Could you check a few things on this model? Use its own coordinates, in mm. A direction names the side the tool comes from. Round coordinates to 2 decimals unless told otherwise and drop trailing zeros. Loops run counter-clockwise (first coordinate to the right, second up) from the corner with the lowest first, then second, coordinate; pieces in that order, holes last. Notation, with made-up numbers: (70, 73.5) -> (78, 73.5) arc R19 cw to (78, 91.5) -> close; hole circle Ø2 at (-1.5, -37.75). An arc over 180 degrees is marked (long way). Put each result on its own line as item: value. Start each with the question number.
1. Imagine slicing it at B-B, the plane x = 11.5. Please give me the cut outline in (y, z).
2. If we mould it in two halves opening along X, with no side actions, what happens to faces 4 (the flat face through (-21, 0, -54)), 5 (the flat face through (-12, 0, 7)), 6 (the flat face through (-28, 0, 9))? For each: pulls with the +X half, pulls with the -X half, needs draft (parallel to the pull), parting line crosses it, or undercut.
3. I'm going to push flat-ended pins straight in: P1, Ø5, axis at x = -24, y = -7, coming from the -Z side; P2, Ø3.5, axis at x = 24, y = 7, coming from the +Z side; P3, Ø1.8, axis at x = -11.5, y = 0, coming from the +Z side; P4, Ø4.5, axis at x = 0, y = 1.5, coming from the -Z side. Where does each tip first touch, or does it pass through?
4. Imagine slicing it at D-D, the plane z = -50. Please give me the cut outline in (x, y).
5. Imagine slicing it at C-C, the plane z = -4. Please give me the cut outline in (x, y), and give its area (3 significant figures).
6. Imagine slicing it at A-A, the plane y = -7. Please give me the cut outline in (x, z), and give its area (3 significant figures).
7. I need wall thicknesses on line 1 (Y direction, x = -24, z = 9.5); line 2 (X direction, y = -1.75, z = 3.5); line 3 (Z direction, x = 16, y = 6). Which ranges of each line are inside material? Lowest first, please. Write a range as [from, to].
8. Which directions (+Z, -Z, +X, -X, +Y, -Y) give clear straight access to the entire face, cutting with the end or side of a thin tool? Please do faces 1 (the flat face through (0, 0, 13)), 2 (the cylindrical face through (-13, 0, 8)), 3 (the cylindrical face through (-0.943, -4.247, -20.39)).
```python
from build123d import *

# Parameters (mm, degrees)
SKETCH_4_R               = 3
EXTRUDE_1_DEPTH          = 54
CUT_EXTRUDE_1_DEPTH      = 63.657800791
SKETCH_6_R               = 4
CUT_EXTRUDE_2_DEPTH      = 4.5
SKETCH_7_R               = 2.25
CUT_EXTRUDE_3_DEPTH      = 21.5
EXTRUDE_2_DEPTH          = 54
SKETCH_9_R               = 2.5
CUT_EXTRUDE_4_DEPTH      = 5
SKETCH_10_R              = 2.5
CUT_EXTRUDE_5_DEPTH      = 5
SKETCH_11_R              = 4.35
CUT_EXTRUDE_6_DEPTH      = 46.5
SKETCH_12_R              = 1.5
CUT_EXTRUDE_7_DEPTH      = 3
SKETCH_13_R              = 1.5
EXTRUDE_4_DEPTH          = 3
SKETCH_14_R              = 1.5
CUT_EXTRUDE_8_DEPTH      = 6
CUT_EXTRUDE_9_DEPTH      = 3
EXTRUDE_START            = 5
SKETCH_16_W              = 56
SKETCH_16_H              = 22
EXTRUDE_5_DEPTH          = 8
SKETCH_18_R              = 3
EXTRUDE_6_DEPTH          = 67
SKETCH_19_R              = 4.35
EXTRUDE_7_DEPTH          = 59.5
SKETCH_20_R              = 2
CUT_EXTRUDE_10_DEPTH     = 8
MIRROR_4_COPY_1_SKETCH_R = 2
MIRROR_4_COPY_1_DEPTH    = 8
CUT_EXTRUDE_START        = -3
SKETCH_21_R              = 1.5
CUT_EXTRUDE_11_DEPTH     = 3
SKETCH_22_R              = 1.5
CUT_EXTRUDE_12_DEPTH     = 3


with BuildPart() as part:
    # 草图4 → 凸台-拉伸1 (new body)
    with BuildSketch(Plane.XY):
        Polygon((-14.75, -7), (-16.25, -7), (-16.25, -6.5), (-20.75, -6.5), (-20.75, -7), (-22.25, -7), (-22.25, -11), (-20.75, -11), (-20.75, -13), (-29, -13), (-29, 13), (-23, 13), (-20.6, 10.6), (-19.1, 10.6), (-16.7, 13), (0, 13), (0, -13), (-16.25, -13), (-16.25, -11), (-14.75, -11), align=None)
        with Locations((-20.5, 0)):
            Circle(SKETCH_4_R, mode=Mode.SUBTRACT)
    extrude(amount=-EXTRUDE_1_DEPTH)

    # 草图5 → 切除-拉伸1 (cut, through all)
    with BuildSketch(Plane.XY):
        Polygon((-5.5, -12), (-4.5, -12), (-4.5, -13), (-2.25, -13), (-2.25, -12), (-1.25, -12), (-1.25, -10), (-5.5, -10), align=None)
    cut_extrude_1 = extrude(amount=-CUT_EXTRUDE_1_DEPTH, mode=Mode.SUBTRACT)

    # 镜向1: 切除-拉伸1 across plane
    add(cut_extrude_1.mirror(Plane.ZX), mode=Mode.SUBTRACT)

    # 草图6 → 切除-拉伸2 (cut)
    with BuildSketch(Plane(origin=(0, 13, 0), x_dir=(-1, 0, 0), z_dir=(0, 1, 0))):
        with Locations(Location((11.5, -25, 0), (0, 0, 90))):
            Circle(SKETCH_6_R)
        with Locations(Location((11.5, -5, 0), (0, 0, 90))):
            Circle(SKETCH_6_R)
    extrude(amount=-CUT_EXTRUDE_2_DEPTH, mode=Mode.SUBTRACT)

    # 草图7 → 切除-拉伸3 (cut)
    with BuildSketch(Plane(origin=(0, 8.5, 0), x_dir=(1, 0, 0), z_dir=(0, 1, 0))):
        with Locations(Location((-11.5, 25, 0), (0, 0, 270))):
            Circle(SKETCH_7_R)
        with Locations(Location((-11.5, 5, 0), (0, 0, 270))):
            Circle(SKETCH_7_R)
    extrude(amount=-CUT_EXTRUDE_3_DEPTH, mode=Mode.SUBTRACT)

    # 镜向2: part across plane


with BuildPart() as part_1:
    add(part.part)
    add(part.part.mirror(Plane(origin=(0, 0, 0), x_dir=(0, 0, 1), z_dir=(1, 0, 0))))

    # 草图8 → 凸台-拉伸2 (add)
    with BuildSketch(Plane.XY):
        Polygon((16.7, 13), (23, 13), (20.6, 10.6), (19.1, 10.6), align=None)
    extrude(amount=-EXTRUDE_2_DEPTH)

    # 草图9 → 切除-拉伸4 (cut)
    with BuildSketch(Plane(origin=(0, 13, 0), x_dir=(1, 0, 0), z_dir=(0, 1, 0))):
        with Locations(Location((18, 46.5, 0), (0, 0, 270))):
            Circle(SKETCH_9_R)
        with Locations(Location((18, 11, 0), (0, 0, 270))):
            Circle(SKETCH_9_R)
    extrude(amount=-CUT_EXTRUDE_4_DEPTH, mode=Mode.SUBTRACT)

    # 草图10 → 切除-拉伸5 (cut)
    with BuildSketch(Plane(origin=(29, 0, 0), x_dir=(0, 0, -1), z_dir=(1, 0, 0))):
        with Locations((11, 8)):
            Circle(SKETCH_10_R)
        with Locations((38.5, 8)):
            Circle(SKETCH_10_R)
    extrude(amount=-CUT_EXTRUDE_5_DEPTH, mode=Mode.SUBTRACT)

    # 草图11 → 切除-拉伸6 (cut)
    with BuildSketch(Plane.XY):
        Circle(SKETCH_11_R)
    extrude(amount=-CUT_EXTRUDE_6_DEPTH, mode=Mode.SUBTRACT)

    # 草图12 → 切除-拉伸7 (cut)
    with BuildSketch(Plane(origin=(0, 0, -54), x_dir=(-1, 0, 0), z_dir=(0, 0, -1))):
        with Locations((-11.5, 0)):
            Circle(SKETCH_12_R)
        with BuildLine():
            Line((11.75, 1.5), (11.25, 1.5))
            ThreePointArc((11.25, 1.5), (9.75, 0), (11.25, -1.5))
            Line((11.25, -1.5), (11.75, -1.5))
            ThreePointArc((11.75, -1.5), (13.25, 0), (11.75, 1.5))
        make_face()
    extrude(amount=-CUT_EXTRUDE_7_DEPTH, mode=Mode.SUBTRACT)

    # 草图13 → 凸台-拉伸4 (add)
    with BuildSketch(Plane(origin=(0, 0, -51), x_dir=(-1, 0, 0), z_dir=(0, 0, -1))):
        with Locations((11.5, 0)):
            Circle(SKETCH_13_R)
        with Locations((-11.5, 0)):
            Circle(SKETCH_13_R)
    extrude(amount=-EXTRUDE_4_DEPTH)

    # 草图14 → 切除-拉伸8 (cut)
    with BuildSketch(Plane.XZ.offset(13)):
        with Locations(Location((-11.5, -15, 0), (0, 0, 270))):
            Circle(SKETCH_14_R)
        with Locations(Location((11.5, -15, 0), (0, 0, 270))):
            Circle(SKETCH_14_R)
    extrude(amount=-CUT_EXTRUDE_8_DEPTH, mode=Mode.SUBTRACT)

    # 草图15 → 切除-拉伸9 (cut)
    with BuildSketch(Plane.XZ.offset(13)):
        with BuildLine():
            Line((-11.75, -13.5), (-11.25, -13.5))
            ThreePointArc((-11.25, -13.5), (-9.75, -15), (-11.25, -16.5))
            Line((-11.25, -16.5), (-11.75, -16.5))
            ThreePointArc((-11.75, -16.5), (-13.25, -15), (-11.75, -13.5))
        make_face()
    extrude(amount=-CUT_EXTRUDE_9_DEPTH, mode=Mode.SUBTRACT)


with BuildPart() as body_2:
    # 草图16 → 凸台-拉伸5 (new body)
    with BuildSketch(Plane.XY.offset(EXTRUDE_START)):
        Rectangle(SKETCH_16_W, SKETCH_16_H)
    extrude(amount=EXTRUDE_5_DEPTH)

    # 草图18 → 凸台-拉伸6 (add)
    with BuildSketch(Plane.XY.offset(13)):
        with Locations((20.5, 0)):
            Circle(SKETCH_18_R)
        with Locations((-20.5, 0)):
            Circle(SKETCH_18_R)
    extrude(amount=-EXTRUDE_6_DEPTH)

    # 草图19 → 凸台-拉伸7 (add)
    with BuildSketch(Plane.XY.offset(13)):
        Circle(SKETCH_19_R)
    extrude(amount=-EXTRUDE_7_DEPTH)

    # 草图20 → 切除-拉伸10 (cut)
    with BuildSketch(Plane.XY.offset(13)):
        with Locations((-24, 7)):
            Circle(SKETCH_20_R)
    cut_extrude_10 = extrude(amount=-CUT_EXTRUDE_10_DEPTH, mode=Mode.SUBTRACT)

    # 镜向3: 切除-拉伸10 across plane
    add(cut_extrude_10.mirror(Plane.ZX), mode=Mode.SUBTRACT)

    # 镜向4: 切除-拉伸10 across plane
    add(cut_extrude_10.mirror(Plane(origin=(0, 0, 0), x_dir=(0, 0, 1), z_dir=(1, 0, 0))), mode=Mode.SUBTRACT)

    # 镜向4 copy 1 sketch → 镜向4 copy 1 (cut)
    with BuildSketch(Plane(origin=(0, 0, 13), x_dir=(-1, 0, 0), z_dir=(0, 0, 1))):
        with Locations((-24, 7)):
            Circle(MIRROR_4_COPY_1_SKETCH_R)
    extrude(amount=-MIRROR_4_COPY_1_DEPTH, mode=Mode.SUBTRACT)

    # 草图21 → 切除-拉伸11 (cut)
    with BuildSketch(Plane.XY.offset(13).offset(CUT_EXTRUDE_START)):
        with Locations((11.5, 0)):
            Circle(SKETCH_21_R)
        with BuildLine():
            Line((-11.75, 1.5), (-11.25, 1.5))
            ThreePointArc((-11.25, 1.5), (-9.75, 0), (-11.25, -1.5))
            Line((-11.25, -1.5), (-11.75, -1.5))
            ThreePointArc((-11.75, -1.5), (-13.25, 0), (-11.75, 1.5))
        make_face()
    extrude(amount=CUT_EXTRUDE_11_DEPTH, mode=Mode.SUBTRACT)

    # 草图22 → 切除-拉伸12 (cut)
    with BuildSketch(Plane.XY.offset(10).offset(CUT_EXTRUDE_START)):
        with Locations((-11.5, 0)):
            Circle(SKETCH_22_R)
        with Locations((11.5, 0)):
            Circle(SKETCH_22_R)
    extrude(amount=CUT_EXTRUDE_12_DEPTH, mode=Mode.SUBTRACT)


solid = body_2.part
```
Entries:
1. outline: (-11, 5) -> (11, 5) -> (11, 13) -> (1.5, 13) -> (1.5, 7) -> (-1.5, 7) -> (-1.5, 13) -> (-11, 13) -> close
2. face 4: needs draft
2. face 5: undercut
2. face 6: pulls with the -X half
3. P1: z = 5
3. P2: through
3. P3: z = 7
3. P4: z = -46.5
4. outline: circle Ø6 at (-20.5, 0); circle Ø6 at (20.5, 0)
5. outline: circle Ø6 at (-20.5, 0); circle Ø8.7 at (0, 0); circle Ø6 at (20.5, 0)
5. area: 116 mm^2
6. outline: (-28, 5) -> (-26, 5) -> (-26, 13) -> (-28, 13) -> close; (-22, 5) -> (22, 5) -> (22, 13) -> (-22, 13) -> close; (26, 5) -> (28, 5) -> (28, 13) -> (26, 13) -> close
6. area: 384 mm^2
7. line 1: [-11, -9], [-5, 5], [9, 11]
7. line 2: [-22.94, -18.06], [-3.98, 3.98], [18.06, 22.94]
7. line 3: [5, 13]
8. face 1: +Z, +X, -X, +Y, -Y
8. face 2: +Z
8. face 3: -Z
